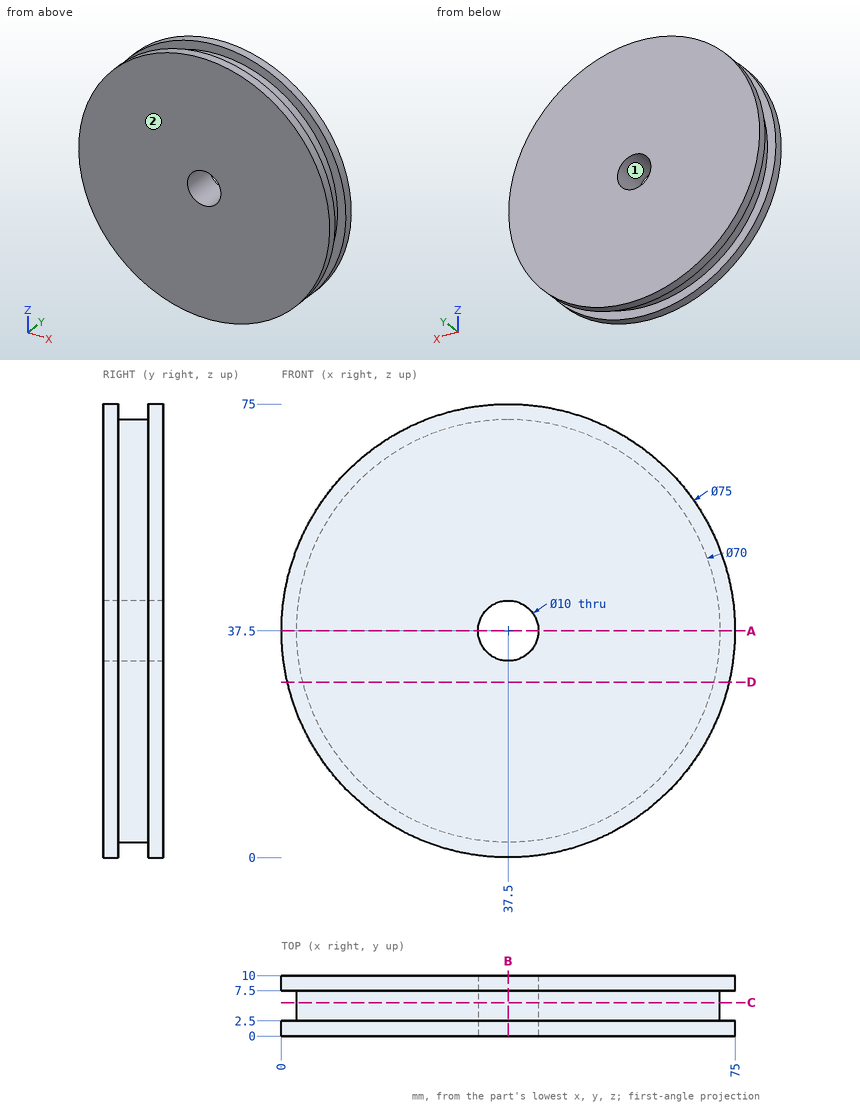
Geometry: see drawing. Coordinates: mm, zero at the bounding-box minimum. Coordinates: 2 decimals unless noted, no trailing zeros. Loops run counter-clockwise (first coordinate to the right, second up) from the corner with the lowest first, then second, coordinate; pieces in that order, holes last. Notation, with made-up numbers: (42, 44) - (51, 44) arc R23 ccw to (51, 83) - close; hole circle Ø1 at (48.25, 40). An arc over 180 degrees is marked (long way). Answer as CSV lines item,"result".
1. Section A-A (z = 37.5). Return loops of the section in (x, y).
Established:
outline,"(0, 0) - (32.5, 0) - (32.5, 10) - (0, 10) - (0, 7.5) - (2.5, 7.5) - (2.5, 2.5) - (0, 2.5) - close; (42.5, 0) - (75, 0) - (75, 2.5) - (72.5, 2.5) - (72.5, 7.5) - (75, 7.5) - (75, 10) - (42.5, 10) - close"
2. Mould query, pull axis X, two halves, no side actions, for the marked faces 1 and 2. Classes: released by +X, released by -X, zero draft, split by the parting line, or undercut.
Established:
face 1,"undercut"
face 2,"zero draft"
3. Section D-D (z = 29). Return loops of the section in (x, y), then the cut area to 3 significant figures.
Established:
outline,"(0.98, 0) - (74.02, 0) - (74.02, 2.5) - (71.45, 2.5) - (71.45, 7.5) - (74.02, 7.5) - (74.02, 10) - (0.98, 10) - (0.98, 7.5) - (3.55, 7.5) - (3.55, 2.5) - (0.98, 2.5) - close"
area,"705 mm2"
4. Contact query for flat-ended pins moving along their axis: pin 1 (1.5 mm diameter, centred on x = 22, y = 1.5, fed in from -Z); pin 2 (1 mm diameter, centred on y = 5, z = 52.5, fed in from +X); pin 3 (1 mm diameter, centred on x = 23.5, y = 2.5, fed in from -Z); pin 4 (8 mm diameter, centred on x = 37.5, z = 37.5, fed in from +Y). Output: stop coordinate, or through.
Established:
pin 1,"stops at z = 3.02"
pin 2,"stops at x = 69.36"
pin 3,"stops at z = 2.51"
pin 4,"passes through"
5. Section B-B (x = 37.5). Return loops of the section in (y, z).
Established:
outline,"(0, 0) - (2.5, 0) - (2.5, 2.5) - (7.5, 2.5) - (7.5, 0) - (10, 0) - (10, 32.5) - (0, 32.5) - close; (0, 42.5) - (10, 42.5) - (10, 75) - (7.5, 75) - (7.5, 72.5) - (2.5, 72.5) - (2.5, 75) - (0, 75) - close"
6. Section C-C (y = 5.5). Return loops of the section in (x, z), then the cut area to 3 significant figures.
Established:
outline,"circle Ø70 at (37.5, 37.5); hole circle Ø10 at (37.5, 37.5)"
area,"3,770 mm2"
7. Ray query, line 1 (X direction, y = 4.25, z = 37.5); line 2 (X direction, y = 8, z = 37.5); line 3 (Y direction, x = 64, z = 12). Return the intervals inside material, ascending.
Established:
line 1,"x = 2.5 to 32.5, 42.5 to 72.5"
line 2,"x = 0 to 32.5, 42.5 to 75"
line 3,"y = 0 to 2.5, 7.5 to 10"
